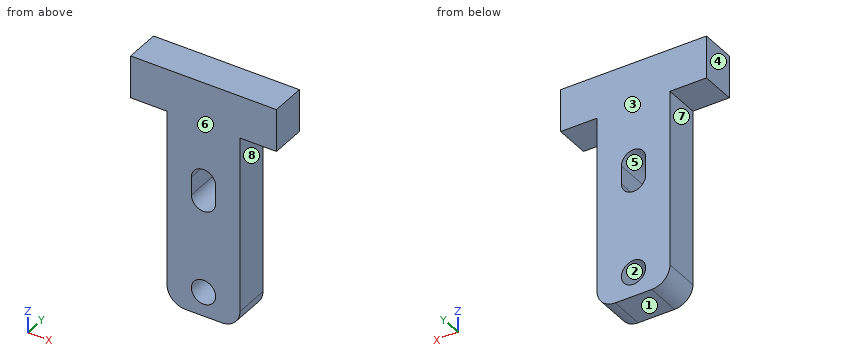
from build123d import *

# Parameters (mm, degrees)
SKETCH1_R           = 2
BOSS_EXTRUDE1_DEPTH = 5.8


with BuildPart() as part:
    # Sketch1 → Boss-Extrude1 (new body)
    with BuildSketch(Plane(origin=(0, 0, 0), x_dir=(1, 0, 0), z_dir=(0, 1, 0))):
        with BuildLine():
            Line((6, -18.624423913), (12, -18.624423913))
            Line((12, -18.624423913), (12, -25.624423913))
            Line((12, -25.624423913), (-12, -25.624423913))
            Line((-12, -25.624423913), (-12, -18.624423913))
            Line((-12, -18.624423913), (-6, -18.624423913))
            Line((-6, -18.624423913), (-6, 10.375576087))
            ThreePointArc((-6, 10.375576087), (-5.121320344, 12.496896431), (-3, 13.375576087))
            Line((-3, 13.375576087), (3, 13.375576087))
            ThreePointArc((3, 13.375576087), (5.121320344, 12.496896431), (6, 10.375576087))
            Line((6, 10.375576087), (6, -18.624423913))
        make_face()
        with Locations(Location((0, 9.375576087, 0), (0, 0, 270))):
            Circle(SKETCH1_R, mode=Mode.SUBTRACT)
        with BuildLine():
            Line((-2, -9.124423913), (-2, -6.124423913))
            ThreePointArc((-2, -6.124423913), (0, -4.124423913), (2, -6.124423913))
            Line((2, -6.124423913), (2, -9.124423913))
            ThreePointArc((2, -9.124423913), (0, -11.124423913), (-2, -9.124423913))
        make_face(mode=Mode.SUBTRACT)
    extrude(amount=BOSS_EXTRUDE1_DEPTH)


solid = part.part
Read the model definition and answer for the solid it produces. Units are mm, in the model's axes. Face numbers are marked on the shaded views. A direction names the side the tool comes from. Coordinates: 2 decimals unless noted, no trailing zeros. Order: outer loops, then holes, each group sorted by start corner. A loop starts at its lowest first (then second) coordinate and runs counter-clockwise, first axis right, second up. Notation, with made-up numbers: M 21,18.25 L 30,18.25 A18 ccw 30,26.25 Z; hole C -5,34.5 d1. An arc over 180 degrees is marked long. Put each result on its own line as item: value. Start each with the question number.
Item 1: For the marked faces 4, 5, 6, 7 and 8, determine the directions among +Z, -Z, +X, -X, +Y, -Y from which every point of the face is accessible in a straight line to the end or side of a thin tool.
Item 2: The mould has two halves that part along Z. Classify the marked faces 1, 2 and 3: +Z half, -Z half, draft (parallel to the pull), parting line (faces both ways), or undercut.
Item 3: Section B-B, the plane x = 0 is taken. Determine the outline of the cut face in (y, z), plus the area to 3 significant figures.
Item 4: Given pin 1 Ø3 at (y, z) = (3, 11) entering from -X; pin 2 Ø4 at (x, z) = (-3, 5.5) entering from -Y; pin 3 Ø2.5 at (y, z) = (3.5, 7.5) entering from +X; pin 4 Ø1.7 at (x, y) = (-7.5, 4) entering from -Z, each flat-ended and moving along its own axis, determine where each tip first touches the part or whether it passes through.
Item 5: Consider probe 1 along X at (y, z) = (3.4, 8.5); probe 2 along X at (y, z) = (4.25, 18.5); probe 3 along Z at (x, y) = (8.5, 3.75). Determine where each line is inside the solid, lowest interval first. Write a range as [from, to].
Item 6: Section D-D, the plane z = 17 is taken. Determine the outline of the cut face in (x, y), plus the area to 3 significant figures.
Item 7: Section A-A, the plane y = 4.2 is taken. Determine the outline of the cut face in (x, z).
Item 8: Section C-C, the plane z = -10 is taken. Determine the outline of the cut face in (x, y), plus the area to 3 significant figures.
Computed:
1. face 4: +Z, -Z, -X, +Y, -Y
1. face 5: +Y, -Y
1. face 6: +Z, -Z, +X, -X, -Y
1. face 7: -Z, -X, +Y, -Y
1. face 8: -Z, +X, +Y, -Y
2. face 1: -Z half
2. face 2: undercut
2. face 3: draft
3. outline: M 0,-13.38 L 5.8,-13.38 L 5.8,-11.38 L 0,-11.38 Z; M 0,-7.38 L 5.8,-7.38 L 5.8,4.12 L 0,4.12 Z; M 0,11.12 L 5.8,11.12 L 5.8,25.62 L 0,25.62 Z
3. area: 162 mm2
4. pin 1: stops at x = -6
4. pin 2: stops at y = 0
4. pin 3: stops at x = 6
4. pin 4: stops at z = 18.62
5. probe 1: x = [-6, -2], [2, 6]
5. probe 2: x = [-6, 6]
5. probe 3: z = [18.62, 25.62]
6. outline: M -6,0 L 6,0 L 6,5.8 L -6,5.8 Z
6. area: 69.6 mm2
7. outline: M -12,18.62 L -6,18.62 L -6,-10.38 A3 ccw -3,-13.38 L 3,-13.38 A3 ccw 6,-10.38 L 6,18.62 L 12,18.62 L 12,25.62 L -12,25.62 Z; hole C 0,-9.38 d4; hole M -2,6.12 A2 ccw 2,6.12 L 2,9.12 A2 ccw -2,9.12 Z
8. outline: M -6,0 L -1.9,0 L -1.9,5.8 L -6,5.8 Z; M 1.9,0 L 6,0 L 6,5.8 L 1.9,5.8 Z
8. area: 47.6 mm2
